Here's how the part is built. I have some questions about the finished solid (model axes, mm). Round coordinates to 2 decimals unless told otherwise and drop trailing zeros. Write each loop counter-clockwise with the first axis right and the second up, starting at its lowest first coordinate (ties: lowest second). Pieces come first, ordered by that corner, then holes. Notation, with made-up numbers: (-11, 66.5) - (15, 66.5) arc R9 cw to (15, 77.5) - close; hole circle Ø1 at (-20, -39.5). An arc over 180 degrees is marked (long way). Write item = value, one per line. Start each with the question number.
Item 1: If we section it at B-B (x = 28.5): Please give me the cut outline in (y, z), and give its area (3 significant figures).
Item 2: If we section it at A-A (z = 0.05): Please give me the cut outline in (x, y).
Item 3: If I drill on line 1 along Y through (x, z) = (48.5, 0.05); line 2 along Y through (x, z) = (18.5, 0.05), over which ranges is the centre line in solid material (lowest first)? Write a range as [from, to].
Item 4: If we section it at C-C (y = -7.2): Please give me the cut outline in (x, z), and give its area (3 significant figures).
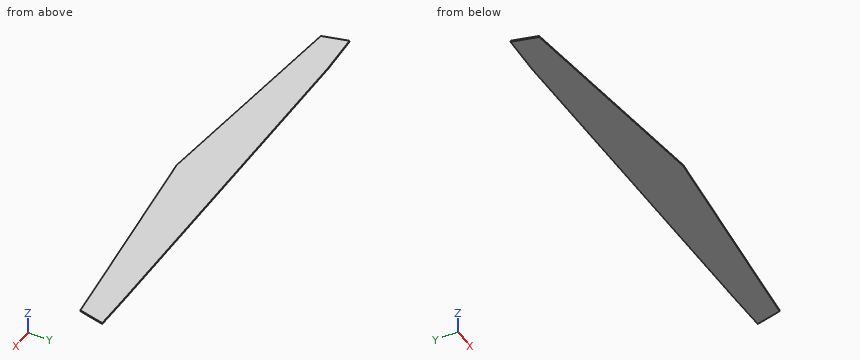
```python
from build123d import *

# Parameters (mm, degrees)
SALIENTE_EXTRUIR1_DEPTH = 0.1


with BuildPart() as part:
    # Model → Saliente-Extruir1 (new body)
    with BuildSketch(Plane.XY):
        with BuildLine():
            Line((47.900286295, -3.880714535), (15.900286295, -3.880714535))
            Line((15.900286295, -3.880714535), (12.202555869, -4.052676889))
            ThreePointArc((12.202555869, -4.052676889), (12.48180991, -5.167779291), (12.778578315, -6.278348831))
            Line((12.778578315, -6.278348831), (31.925658705, -8.308398583))
            Line((31.925658705, -8.308398583), (50.990379009, -6.152892242))
            ThreePointArc((50.990379009, -6.152892242), (51.263698747, -5.03797547), (51.52136497, -3.919337367))
            Line((51.52136497, -3.919337367), (47.900286295, -3.880714535))
        make_face()
    extrude(amount=SALIENTE_EXTRUIR1_DEPTH)


solid = part.part
```
Reply:
q1.outline = (-7.95, 0) - (-3.88, 0) - (-3.88, 0.1) - (-7.95, 0.1) - close
q1.area = 0.406 mm2
q2.outline = (12.2, -4.05) arc R73.04 ccw to (12.78, -6.28) - (31.93, -8.31) - (50.99, -6.15) arc R81.9 ccw to (51.52, -3.92) - (47.9, -3.88) - (15.9, -3.88) - close
q3.line_1 = [-6.43, -3.89]
q3.line_2 = [-6.88, -3.88]
q4.outline = (21.47, 0) - (41.73, 0) - (41.73, 0.1) - (21.47, 0.1) - close
q4.area = 2.03 mm2
